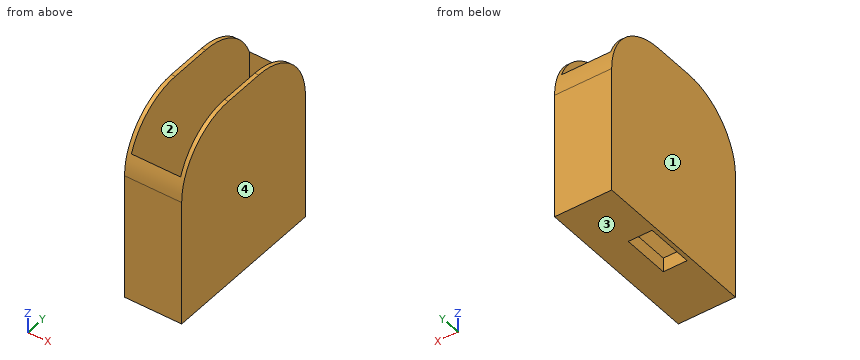
```python
from build123d import *

# Parameters (mm, degrees)
F1_DEPTH    = 1.8
F0_W        = 7.2
F0_H        = 21.2
F2_DEPTH    = 24
F3_T1_DEPTH = 47.2


# Not quite as in the source:
# - a fillet or chamfer that OpenCascade refuses, or shapes differently, is made with other operations: its cross-section is extruded or revolved along the edge and cut away or added


with BuildPart() as f1:
    # F0 (on Top) → F1 (new body)
    with BuildSketch(Plane.XY):
        Polygon((0, 7.1), (0, 0), (6.2, 0), (6.2, 20.2), (0, 20.2), (0, 13.1), (3, 13.1), (3, 10.1), (3, 7.1), align=None)
    extrude(amount=F1_DEPTH)

    # F0 (on Top) → F2 (join)
    with BuildSketch(Plane.XY):
        with Locations((3.1, 10.1)):
            Rectangle(F0_W, F0_H)
        Polygon((6.2, 0), (0, 0), (0, 7.1), (0, 10.1), (0, 13.1), (0, 20.2), (6.2, 20.2), align=None, mode=Mode.SUBTRACT)
    extrude(amount=F2_DEPTH)

    # F3: fillet of radius 8 on 2 edges, made by hand

    # F3_s2 → F3_t1 (cut)
    with BuildSketch(Plane.YZ.offset(-20.5)):
        with BuildLine():
            ThreePointArc((7.5, 24), (1.8431457505, 21.6568542495), (-0.5, 16))
            Line((-0.5, 16), (-0.5, 24))
            Line((-0.5, 24), (7.5, 24))
        make_face()
        with BuildLine():
            ThreePointArc((12.7, 24), (18.3568542495, 21.6568542495), (20.7, 16))
            Line((20.7, 16), (20.7, 24))
            Line((20.7, 24), (12.7, 24))
        make_face()
    extrude(amount=F3_T1_DEPTH, mode=Mode.SUBTRACT)


solid = f1.part
```
Part model, mm, in its own coordinate system. Face numbers are marked on the shaded views. Round coordinates to 2 decimals unless told otherwise and drop trailing zeros. Write each loop counter-clockwise with the first axis right and the second up, starting at its lowest first coordinate (ties: lowest second). Pieces come first, ordered by that corner, then holes.
Item 1: Two-plate mould, pull along X, no slides. Class the marked faces 1, 2, 3 and 4: +X half, -X half, draft (parallel to the pull), parting line (faces both ways), or undercut.
Results:
face 1: -X half
face 2: undercut
face 3: draft
face 4: +X half
Item 2: Drop a flat-ended pin along its axis: pin 1 Ø4 at (x, y) = (4.5, 17) entering from +Z. Give the stop position or say it passes through.
Results:
pin 1: stops at z = 23.31
Item 3: Probe L1, parallel to Y at x = 4, z = 13.75; L2, parallel to X at y = 5.5, z = 6; L3, parallel to Z at x = 4.5, y = 6. List the from-to ranges inside material, lowest first.
Results:
L1: y = -0.5 to 0, 20.2 to 20.7
L2: x = -0.5 to 0, 6.2 to 6.7
L3: z = 0 to 1.8
Item 4: Cut at A-A, the plane x = 2.5. Give the cut face in (y, z).
Results:
outline: (-0.5, 0) - (7.1, 0) - (7.1, 1.8) - (0, 1.8) - (0, 18.78) arc R8 ccw to (-0.5, 16) - close; (13.1, 0) - (20.7, 0) - (20.7, 16) arc R8 ccw to (20.2, 18.78) - (20.2, 1.8) - (13.1, 1.8) - close
Item 5: Cut at B-B, the plane y = 8.75. Give the cut face in (x, z), plus the area to 3 significant figures.
Results:
outline: (-0.5, 0) - (0, 0) - (0, 24) - (-0.5, 24) - close; (3, 0) - (6.7, 0) - (6.7, 24) - (6.2, 24) - (6.2, 1.8) - (3, 1.8) - close
area: 29.8 mm2
Item 6: Cut at C-C, the plane z = 19.75. Give the cut face in (x, y).
Results:
outline: (-0.5, 0.43) - (0, 0.43) - (0, 19.77) - (-0.5, 19.77) - close; (6.2, 0.43) - (6.7, 0.43) - (6.7, 19.77) - (6.2, 19.77) - close
Item 7: Cut at D-D, the plane z = 13.75. Give the cut face in (x, y), plus the area to 3 significant figures.
Results:
outline: (-0.5, -0.5) - (6.7, -0.5) - (6.7, 20.7) - (-0.5, 20.7) - close; hole (0, 0) - (6.2, 0) - (6.2, 20.2) - (0, 20.2) - close
area: 27.4 mm2
